```python
from build123d import *

# Parameters (mm, degrees)
F0_W     = 50
F0_H     = 50
F1_DEPTH = 100
F3_DEPTH = 50
F4_W     = 10
F4_H     = 10
F5_DEPTH = 20


with BuildPart() as f1:
    # F0 (on Right) → F1 (new body, symmetric)
    with BuildSketch(Plane.YZ):
        Rectangle(F0_W, F0_H)
    extrude(amount=F1_DEPTH, both=True)

    # F2 (on face) → F3 (cut, through all)
    with BuildSketch(Plane.XZ.offset(25)):
        Polygon((-60, 5), (-60, -5), (0, -5), (0, 5), (80, 5), (80, -5), (70, -5), (70, -25), (100, -25), (100, 25), (-50, 25), (-50, 5), align=None)
    extrude(amount=-F3_DEPTH, mode=Mode.SUBTRACT)

    # F4 (on face) → F5 (cut, through all)
    with BuildSketch(Plane.XY.offset(25)):
        with Locations((-55, 0)):
            Rectangle(F4_W, F4_H)
    extrude(amount=-F5_DEPTH, mode=Mode.SUBTRACT)


solid = f1.part
```
Geometry: final body of the model. Coordinates: model frame, mm. A direction names the side the tool comes from. Coordinates: 2 decimals unless noted, no trailing zeros. Order: outer loops, then holes, each group sorted by start corner. A loop starts at its lowest first (then second) coordinate and runs counter-clockwise, first axis right, second up. Notation, with made-up numbers: (-38.75, 76) - (-11.75, 76) arc R22 ccw to (-11.75, 86) - close; hole circle Ø9 at (-12.75, 60.25). An arc over 180 degrees is marked (long way). Write each question's results on one line, items separated by ' | '.
1) Section C-C, the plane y = -20. Return loops of the section in (x, z), plus the area to 3 significant figures.
Results list:
outline: (-100, -25) - (70, -25) - (70, -5) - (80, -5) - (80, 5) - (0, 5) - (0, -5) - (-60, -5) - (-60, 5) - (-50, 5) - (-50, 25) - (-100, 25) - close | area: 5,600 mm^2
2) Section A-A, the plane x = -53. Return loops of the section in (y, z), plus the area to 3 significant figures.
Results list:
outline: (-25, -25) - (25, -25) - (25, -5) - (-25, -5) - close; (-25, 5) - (-5, 5) - (-5, 25) - (-25, 25) - close; (5, 5) - (25, 5) - (25, 25) - (5, 25) - close | area: 1,800 mm^2
3) Pull-direction query (Y, two-part tool) for faces 6 (the flat face through (-55, -5, 15)), 7 (the flat face through (-29, -25, -6)), 8 (the flat face through (-29, 25, -6)); classes: pulls with the +Y half, pulls with the -Y half, needs draft (parallel to the pull), parting line crosses it, or undercut.
Results list:
face 6: undercut | face 7: pulls with the -Y half | face 8: pulls with the +Y half
4) Section D-D, the plane z = 19. Return loops of the section in (x, y).
Results list:
outline: (-100, -25) - (-50, -25) - (-50, -5) - (-60, -5) - (-60, 5) - (-50, 5) - (-50, 25) - (-100, 25) - close
5) Pin query (flat end, axial travel): pin 1 (6 mm diameter, centred on y = -7, z = -13, fed in from +X); pin 2 (5 mm diameter, centred on y = 15, z = 12.5, fed in from +X); pin 3 (8 mm diameter, centred on x = 18.5, y = 9, fed in from +Z). Return the tip coordinate at first contact, or that it passes through.
Results list:
pin 1: x = 70 | pin 2: x = -50 | pin 3: z = 5
6) Set-up query: faces 1 (the flat face through (-55, -15, 5)), 2 (the flat face through (70, 0, -15)), 3 (the flat face through (-55, 5, 15)), 4 (the flat face through (0, 0, 0)), 5 (the flat face through (-50, -15, 15)). Return all of +Z, -Z, +X, -X, +Y, -Y with unobstructed straight access to the full face (end or side cutting, diameter ignored); none if empty.
Results list:
face 1: +Y, -Y | face 2: -Z, +X, +Y, -Y | face 3: +Z, +X | face 4: +Z, +Y, -Y | face 5: +Z, +X, +Y, -Y
7) Line query: line 1 (Z direction, x = -2, y = -16.5); line 2 (X direction, y = 15.5, z = -17.5); line 3 (X direction, y = 13, z = 11). Output: solid intervals per line, ascending. Write a range as from..to.
Results list:
line 1: -25..-5 | line 2: -100..70 | line 3: -100..-50
8) Section B-B, the plane z = 2. Return loops of the section in (x, y).
Results list:
outline: (-100, -25) - (-60, -25) - (-60, 25) - (-100, 25) - close; (0, -25) - (80, -25) - (80, 25) - (0, 25) - close
